For this review, take the finished solid that the model builds, in its own axes (mm). Face numbers are marked on the shaded views. A direction names the side the tool comes from. Round coordinates to 2 decimals unless told otherwise and drop trailing zeros. Loops run counter-clockwise (first coordinate to the right, second up) from the corner with the lowest first, then second, coordinate; pieces in that order, holes last. Notation, with made-up numbers: M -18.75,-36 L 6.25,-36 A17 ccw 6.25,-17 Z; hole C 22,-18 d3. An arc over 180 degrees is marked long. Write item = value, one per line. Start each with the question number.
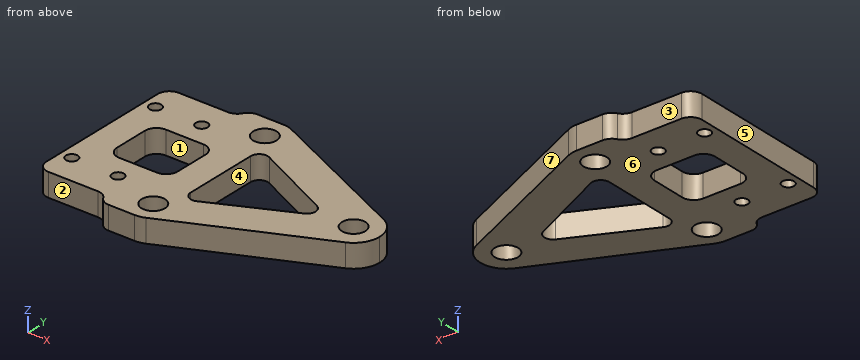
```python
from build123d import *

# Parameters (mm, degrees)
SKETCH_1_W          = 48
SKETCH_1_H          = 32
EXTRUDE_1_DEPTH     = 4
SKETCH_2_R          = 2.025
SKETCH_2_R_2        = 1.025
CUT_EXTRUDE_1_DEPTH = 30.8
CUT_EXTRUDE_2_DEPTH = 10
SKETCH_5_W          = 12
SKETCH_5_H          = 2
CUT_EXTRUDE_3_DEPTH = 10
FILLET_1_R          = 2
CUT_EXTRUDE_4_DEPTH = 10
FILLET_2_R          = 1.5
SKETCH_7_W          = 10.5
SKETCH_7_H          = 10
CUT_EXTRUDE_5_DEPTH = 10
FILLET_3_R          = 2


with BuildPart() as part:
    # 草图1 → 凸台-拉伸1 (new body)
    with BuildSketch(Plane.XY):
        Rectangle(SKETCH_1_W, SKETCH_1_H)
    extrude(amount=EXTRUDE_1_DEPTH)

    # 草图2 → 切除-拉伸1 (cut)
    with BuildSketch(Plane(origin=(0, 0, 0), x_dir=(-1, 0, 0), z_dir=(0, 0, -1))):
        with Locations((-19.5, 0)):
            Circle(SKETCH_2_R)
        with Locations((5.5, -12)):
            Circle(SKETCH_2_R)
        with Locations((5.5, 12)):
            Circle(SKETCH_2_R)
        with Locations((14, -9)):
            Circle(SKETCH_2_R_2)
        with Locations((22, -9)):
            Circle(SKETCH_2_R_2)
    cut_extrude_1 = extrude(amount=-CUT_EXTRUDE_1_DEPTH, mode=Mode.SUBTRACT)

    # 草图4 → 切除-拉伸2 (cut)
    with BuildSketch(Plane(origin=(0, 0, 0), x_dir=(-1, 0, 0), z_dir=(0, 0, -1))):
        with BuildLine():
            Line((-21.373826305, 4.091304802), (3.834376618, 15.636715379))
            ThreePointArc((3.834376618, 15.636715379), (4.647609689, 15.908123688), (5.5, 16))
            Line((5.5, 16), (-24, 16))
            Line((-24, 16), (-24, 0))
            ThreePointArc((-24, 0), (-23.286965696, 2.430821017), (-21.373826305, 4.091304802))
        make_face()
    cut_extrude_2 = extrude(amount=-CUT_EXTRUDE_2_DEPTH, mode=Mode.SUBTRACT)

    # 镜向1: 切除-拉伸2 across plane
    add(cut_extrude_2.mirror(Plane.ZX), mode=Mode.SUBTRACT)

    # 草图5 → 切除-拉伸3 (cut)
    with BuildSketch(Plane(origin=(0, 0, 0), x_dir=(-1, 0, 0), z_dir=(0, 0, -1))):
        with Locations((18, -15)):
            Rectangle(SKETCH_5_W, SKETCH_5_H)
        with Locations((18, 15)):
            Rectangle(SKETCH_5_W, SKETCH_5_H)
    extrude(amount=-CUT_EXTRUDE_3_DEPTH, mode=Mode.SUBTRACT)

    # 圆角1
    fillet_1_edges = [part.edges().sort_by_distance(p)[0] for p in [
        (-24, -14, 2),
        (-24, 14, 2),
        (-12, -16, 2),
        (-12, 16, 2),
    ]]
    fillet(fillet_1_edges, radius=FILLET_1_R - 0.0001)  # a hair under: the kernel refuses the full size

    # 草图6 → 切除-拉伸4 (cut)
    with BuildSketch(Plane(origin=(0, 0, 0), x_dir=(-1, 0, 0), z_dir=(0, 0, -1))):
        Polygon((3.5, 8.82153206), (-14.878191792, 0), (3.5, -8.82153206), align=None)
    extrude(amount=-CUT_EXTRUDE_4_DEPTH, mode=Mode.SUBTRACT)

    # 圆角2
    fillet_2_edges = [part.edges().sort_by_distance(p)[0] for p in [
        (-3.5, 8.82153206, 2),
        (-3.5, -8.82153206, 2),
        (14.878191792, 0, 2),
    ]]
    fillet(fillet_2_edges, radius=FILLET_2_R)

    # 镜向2: 切除-拉伸1 across plane
    add(cut_extrude_1.mirror(Plane.ZX), mode=Mode.SUBTRACT)

    # 草图7 → 切除-拉伸5 (cut)
    with BuildSketch(Plane(origin=(0, 0, 0), x_dir=(-1, 0, 0), z_dir=(0, 0, -1))):
        with Locations((13.75, 0)):
            Rectangle(SKETCH_7_W, SKETCH_7_H)
    extrude(amount=-CUT_EXTRUDE_5_DEPTH, mode=Mode.SUBTRACT)

    # 圆角3
    fillet_3_edges = [part.edges().sort_by_distance(p)[0] for p in [
        (-19, 5, 2),
        (-19, -5, 2),
        (-8.5, -5, 2),
        (-8.5, 5, 2),
        (-12, -14, 2),
        (-12, 14, 2),
    ]]
    fillet(fillet_3_edges, radius=FILLET_3_R)


solid = part.part
```
(1) Tool access review of the marked faces 1, 2 and 3: name each direction out of +Z, -Z, +X, -X, +Y, -Y from which nothing blocks a thin tool from reaching the whole face with its end or side.
(2) Wall thickness on L1, parallel to Y at x = -5.5, z = 2.35 (3 decimals); L2, parallel to Y at x = -14, z = 2.2 (3 decimals); L3, parallel to Y at x = -16, z = 0.95: over which ranges is each line inside the solid? List them lowest first.
(3) Add section A-A on x = -14. Write out the cut boundary in (y, z) (3 decimals), and give its area (3 significant figures).
(4) Add section C-C on y = -9. Write out the cut boundary in (x, z) (3 decimals).
(5) Add section D-D on x = 6. Write out the cut boundary in (y, z), and give its area (3 significant figures).
(6) Draft analysis for pull direction X (two halves, no side actions). For the marked faces 4, 5, 6 and 7, state which applies: +X half, -X half, draft (parallel to the pull), parting line (faces both ways), or undercut.
(7) Add section B-B on z = 2.2. Count the separate pieces of the cut face and the enclosed holes in it, and give its area (3 significant figures).
(8) For pin 1 Ø2 at (x, z) = (11, 0.5) entering from -Y; pin 2 Ø1.5 at (y, z) = (-8.5, 1.5) entering from +X; pin 3 Ø1.5 at (y, z) = (12, 3.5) entering from +X, all flat-tipped, find the tip position at first contact; note any pin that passes through.
Answer sheet:
q1.face_1 = +Z, -Z
q1.face_2 = +Z, -Z, -X, -Y
q1.face_3 = +Z, -Z, -X, +Y
q2.L1 = -16 to -14.025, -9.975 to 9.975, 14.025 to 16
q2.L2 = -14 to -10.025, -7.975 to -5, 5 to 7.975, 10.025 to 14
q2.L3 = -14 to -5, 5 to 14
q3.outline = M -14,0 L -10.025,0 L -10.025,4 L -14,4 Z; M -7.975,0 L -5,0 L -5,4 L -7.975,4 Z; M 5,0 L 7.975,0 L 7.975,4 L 5,4 Z; M 10.025,0 L 14,0 L 14,4 L 10.025,4 Z
q3.area = 55.6 mm²
q4.outline = M -24,0 L -23.025,0 L -23.025,4 L -24,4 Z; M -20.975,0 L -15.025,0 L -15.025,4 L -20.975,4 Z; M -12.975,0 L 10.656,0 L 10.656,4 L -12.975,4 Z
q5.outline = M -11.13,0 L -4.26,0 L -4.26,4 L -11.13,4 Z; M 4.26,0 L 11.13,0 L 11.13,4 L 4.26,4 Z
q5.area = 55.0 mm²
q6.face_4 = undercut
q6.face_5 = -X half
q6.face_6 = draft
q6.face_7 = +X half
q7.separate_pieces = 1
q7.enclosed_holes = 9
q7.area = 796 mm²
q8.pin_1 = -9.3
q8.pin_2 = 13.39
q8.pin_3 = 5.74
